Can you work these out from the model? Positions are in its coordinate system, mm. Face numbers are marked on the shaded views. A direction names the side the tool comes from. Give positions to 0.01 mm unless a question says otherwise; leave off trailing zeros. Loops run counter-clockwise (first coordinate to the right, second up) from the corner with the lowest first, then second, coordinate; pieces in that order, holes last. Notation, with made-up numbers: (56.25, 43.25) -> (98.25, 43.25) arc R29 ccw to (98.25, 71.25) -> close; hole circle Ø9 at (88, 3). An arc over 180 degrees is marked (long way). One line per question, with ' | ' between items.
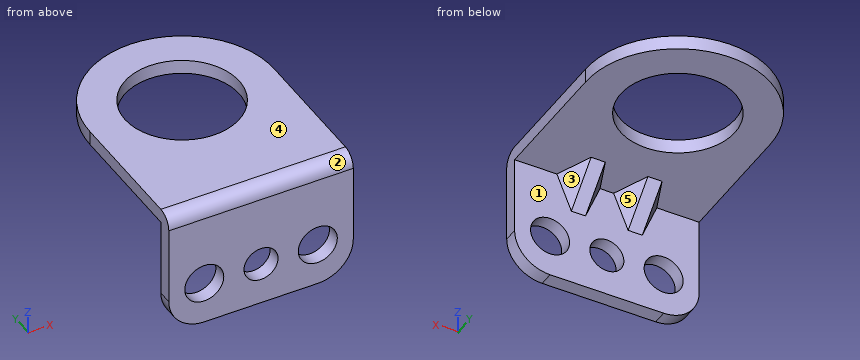
from build123d import *

# Parameters (mm, degrees)
BOSS_EXTRUDE1_DEPTH = 13
SKETCH12_R          = 8.05
BOSS_EXTRUDE2_DEPTH = 2
FILLET3_R           = 2
SKETCH15_R          = 2.4
SKETCH15_R_2        = 2.75
CUT_EXTRUDE1_DEPTH  = 2
FILLET4_R           = 5
RIB1_REACH          = 43.255
SKETCH17_WALL_W     = 91.58167319
SKETCH17_WALL_H     = 2
RIB1_DRAFT_ANGLE    = 30
RIB2_REACH          = 43.255
SKETCH18_WALL_W     = 91.58167319
SKETCH18_WALL_H     = 2
RIB2_DRAFT_ANGLE    = 30


with BuildPart() as part:
    # Sketch1 → Boss-Extrude1 (new, symmetric)
    with BuildSketch(Plane(origin=(0, 0, 0), x_dir=(0, 0, -1), z_dir=(1, 0, 0))):
        Polygon((0, 7.5), (2, 7.5), (2, 2), (18, 2), (18, 0), (0, 0), align=None)
    extrude(amount=BOSS_EXTRUDE1_DEPTH, both=True)

    # Sketch12 → Boss-Extrude2 (add)
    with BuildSketch(Plane(origin=(0, 0, -2), x_dir=(-1, 0, 0), z_dir=(0, 0, -1))):
        with BuildLine():
            Line((13, 20), (13, 7.5))
            Line((13, 7.5), (-13, 7.5))
            Line((-13, 7.5), (-13, 20))
            ThreePointArc((-13, 20), (0, 33), (13, 20))
        make_face()
        with Locations((0, 20)):
            Circle(SKETCH12_R, mode=Mode.SUBTRACT)
    extrude(amount=-BOSS_EXTRUDE2_DEPTH)

    # Fillet3
    fillet3_edges = [part.edges().sort_by_distance(p)[0] for p in [
        (0, 0, 0),
    ]]
    fillet(fillet3_edges, radius=FILLET3_R)

    # Sketch15 → Cut-Extrude1 (cut)
    with BuildSketch(Plane(origin=(0, 2, 0), x_dir=(1, 0, 0), z_dir=(0, 1, 0))):
        with Locations(Location((0, 12, 0), (0, 0, 270))):
            Circle(SKETCH15_R)
        with Locations(Location((8, 12, 0), (0, 0, 270))):
            Circle(SKETCH15_R_2)
        with Locations(Location((-8, 12, 0), (0, 0, 270))):
            Circle(SKETCH15_R_2)
    extrude(amount=-CUT_EXTRUDE1_DEPTH, mode=Mode.SUBTRACT)

    # Fillet4
    fillet4_edges = [part.edges().sort_by_distance(p)[0] for p in [
        (13, 1, -18),
        (-13, 1, -18),
    ]]
    fillet(fillet4_edges, radius=FILLET4_R)

    # Sketch17 wall → Rib1 (add, up to next)
    with BuildSketch(Plane(origin=(4, 4.5, -4.5), x_dir=(0, -0.707106781187, -0.707106781187), z_dir=(0, 0.707106781187, -0.707106781187)), mode=Mode.PRIVATE) as rib1_sk1:
        Rectangle(SKETCH17_WALL_W, SKETCH17_WALL_H)
    rib1_tool1 = extrude(rib1_sk1.sketch, amount=-RIB1_REACH, mode=Mode.PRIVATE) - part.part
    add(rib1_tool1.solids().sort_by_distance((4, 4.5, -4.5))[0])

    # Rib1 draft
    rib1_draft_faces = [part.faces().sort_by_distance(p)[0] for p in [
        (3, 4.146446609, -4.146446609),
        (5, 4.146446609, -4.146446609),
    ]]
    draft(rib1_draft_faces, Plane(origin=(4, 4.5, -4.5), x_dir=(0, -0.707106781187, -0.707106781187), z_dir=(0, 0.707106781187, -0.707106781187)), RIB1_DRAFT_ANGLE)

    # Sketch18 wall → Rib2 (add, up to next)
    with BuildSketch(Plane(origin=(-4, 4.5, -4.5), x_dir=(0, -0.707106781187, -0.707106781187), z_dir=(0, 0.707106781187, -0.707106781187)), mode=Mode.PRIVATE) as rib2_sk1:
        Rectangle(SKETCH18_WALL_W, SKETCH18_WALL_H)
    rib2_tool1 = extrude(rib2_sk1.sketch, amount=-RIB2_REACH, mode=Mode.PRIVATE) - part.part
    add(rib2_tool1.solids().sort_by_distance((-4, 4.5, -4.5))[0])

    # Rib2 draft
    rib2_draft_faces = [part.faces().sort_by_distance(p)[0] for p in [
        (-5, 4.146446609, -4.146446609),
        (-3, 4.146446609, -4.146446609),
    ]]
    draft(rib2_draft_faces, Plane(origin=(-4, 4.5, -4.5), x_dir=(0, -0.707106781187, -0.707106781187), z_dir=(0, 0.707106781187, -0.707106781187)), RIB2_DRAFT_ANGLE)


solid = part.part
Q1. If we section it at C-C (y = 13): Write out the boundary of the cut face in (x, z), plus the area to 3 significant figures.
Entries:
outline: (-13, -2) -> (-3.98, -2) -> (-3.98, 0) -> (-13, 0) -> close; (3.98, -2) -> (13, -2) -> (13, 0) -> (3.98, 0) -> close | area: 36.1 mm²
Q2. On a 3-axis mill with a long thin cutter (end or side, diameter ignored), from which of +Z, -Z, +X, -X, +Y, -Y can I reach the whole of each face in a straight line? I mean the marked faces 1 and 2. Say none if no direction works.
Entries:
face 1: -Z, +Y | face 2: +Z, +X, -X, -Y
Q3. If we mould it in two halves opening along X, with no side actions, what happens to the marked faces 3, 4 and 5? For each: pulls with the +X half, pulls with the -X half, needs draft (parallel to the pull), parting line crosses it, or undercut.
Entries:
face 3: pulls with the +X half | face 4: needs draft | face 5: undercut
Q4. For pin 1 Ø4 at (x, z) = (-7, -9.5) entering from +Y; pin 2 Ø14.5 at (x, y) = (0, 20) entering from -Z, each with a flat end and sliding along its axis, tell me the tip position at first contact or that it passes through.
Entries:
pin 1: y = 2 | pin 2: through
Q5. If we section it at B-B (z = -12): Write out the boundary of the cut face in (x, y), plus the area to 3 significant figures.
Entries:
outline: (-13, 0) -> (-10.75, 0) -> (-10.75, 2) -> (-13, 2) -> close; (-5.25, 0) -> (-2.4, 0) -> (-2.4, 2) -> (-5.25, 2) -> close; (2.4, 0) -> (5.25, 0) -> (5.25, 2) -> (2.4, 2) -> close; (10.75, 0) -> (13, 0) -> (13, 2) -> (10.75, 2) -> close | area: 20.4 mm²
Q6. If I drill on probe 1 along Y at (x, z) = (-11.5, -6.5); probe 2 along Z at (x, y) = (1.5, 9); probe 3 along Y at (x, z) = (0, -0.85), over which ranges is the centre line in solid material (lowest first)? Write a range as from..to.
Entries:
probe 1: 0..2 | probe 2: -2..0 | probe 3: 0.36..11.95, 28.05..33
Q7. If we section it at A-A (x = 0): Write out the boundary of the cut face in (y, z), plus the area to 3 significant figures.
Entries:
outline: (0, -18) -> (2, -18) -> (2, -14.4) -> (0, -14.4) -> close; (0, -9.6) -> (2, -9.6) -> (2, -2) -> (11.95, -2) -> (11.95, 0) -> (2, 0) arc R2 ccw to (0, -2) -> close; (28.05, -2) -> (33, -2) -> (33, 0) -> (28.05, 0) -> close | area: 55.3 mm²
Q8. If we section it at D-D (x = -9.25): Write out the boundary of the cut face in (y, z).
Entries:
outline: (0, -17.84) -> (2, -17.84) -> (2, -14.45) -> (0, -14.45) -> close; (0, -9.55) -> (2, -9.55) -> (2, -2) -> (29.13, -2) -> (29.13, 0) -> (2, 0) arc R2 ccw to (0, -2) -> close
